Source: CAD feature listing. Evaluate the final solid. Frame: model axes, mm. Face numbers are marked on the shaded views. A direction names the side the tool comes from. Round coordinates to 2 decimals unless told otherwise and drop trailing zeros. Loops run counter-clockwise (first coordinate to the right, second up) from the corner with the lowest first, then second, coordinate; pieces in that order, holes last. Notation, with made-up numbers: M 62,73.25 L 75,73.25 A32 ccw 75,112.25 Z; hole C 32.5,75 d11. An arc over 180 degrees is marked long. Answer as a JSON object with one key per item and string values.
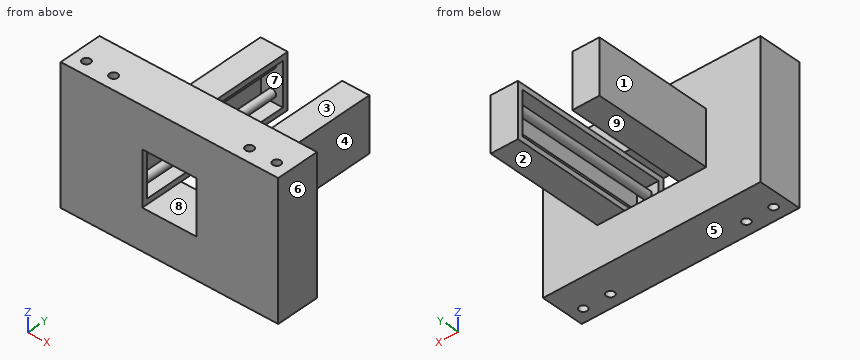
from build123d import *

# Parameters (mm, degrees)
SKETCH1_W           = 400
SKETCH1_H           = 250
BOSS_EXTRUDE1_DEPTH = 80
SKETCH2_R           = 7.5
CUT_EXTRUDE1_DEPTH  = 479.434948556
SKETCH5_W           = 200
SKETCH5_H           = 100
CUT_EXTRUDE2_DEPTH  = 479.434948556
SKETCH8_W           = 100
SKETCH8_H           = 300
BOSS_EXTRUDE2_DEPTH = 50
SKETCH9_W           = 80
SKETCH9_H           = 280
CUT_EXTRUDE3_DEPTH  = 40
SKETCH10_R          = 7.5
BOSS_EXTRUDE3_DEPTH = 280


with BuildPart() as part:
    # Sketch1 → Boss-Extrude1 (new body)
    with BuildSketch(Plane(origin=(0, 0, 0), x_dir=(1, 0, 0), z_dir=(0, 1, 0))):
        with Locations((-200, 125)):
            Rectangle(SKETCH1_W, SKETCH1_H)
    extrude(amount=BOSS_EXTRUDE1_DEPTH)

    # Sketch2 → Cut-Extrude1 (cut, through all)
    with BuildSketch(Plane.XY):
        with Locations((-375, 25)):
            Circle(SKETCH2_R)
        with Locations((-325, 25)):
            Circle(SKETCH2_R)
        with Locations((-75, 25)):
            Circle(SKETCH2_R)
        with Locations((-25, 25)):
            Circle(SKETCH2_R)
    extrude(amount=-CUT_EXTRUDE1_DEPTH, mode=Mode.SUBTRACT)

    # Sketch5 → Cut-Extrude2 (cut, through all)
    with BuildSketch(Plane(origin=(0, 80, 0), x_dir=(1, 0, 0), z_dir=(0, 1, 0))):
        with Locations((-200, 125)):
            Rectangle(SKETCH5_W, SKETCH5_H)
    extrude(amount=-CUT_EXTRUDE2_DEPTH, mode=Mode.SUBTRACT)

    # Sketch8 → Boss-Extrude2 (add)
    with BuildSketch(Plane(origin=(-300, 0, 0), x_dir=(0, 0, -1), z_dir=(1, 0, 0))):
        with Locations((125, 150)):
            Rectangle(SKETCH8_W, SKETCH8_H)
    boss_extrude2 = extrude(amount=BOSS_EXTRUDE2_DEPTH)

    # Sketch9 → Cut-Extrude3 (cut)
    with BuildSketch(Plane(origin=(-250, 0, 0), x_dir=(0, 0, -1), z_dir=(1, 0, 0))):
        with Locations((125, 150)):
            Rectangle(SKETCH9_W, SKETCH9_H)
    cut_extrude3 = extrude(amount=-CUT_EXTRUDE3_DEPTH, mode=Mode.SUBTRACT)

    # Mirror1: Boss-Extrude2, Cut-Extrude3 across plane
    add(boss_extrude2.mirror(Plane.ZY.offset(200)))
    add(cut_extrude3.mirror(Plane.ZY.offset(200)), mode=Mode.SUBTRACT)

    # Sketch10 → Boss-Extrude3 (add)
    with BuildSketch(Plane(origin=(0, 10, 0), x_dir=(1, 0, 0), z_dir=(0, 1, 0))):
        with Locations(Location((-270, 150, 0), (0, 0, 90))):
            Circle(SKETCH10_R)
        with Locations(Location((-270, 100, 0), (0, 0, 90))):
            Circle(SKETCH10_R)
    boss_extrude3 = extrude(amount=BOSS_EXTRUDE3_DEPTH)

    # Mirror2: Boss-Extrude3 across plane
    add(boss_extrude3.mirror(Plane.ZY.offset(200)))


solid = part.part
Item 1: Section B-B on y = 73.5. Return the cut outline in (x, z).
Answer sheet:
{"outline": "M -400,-250 L 0,-250 L 0,0 L -400,0 Z; C -270,-150 d15; C -270,-100 d15; C -130,-150 d15; C -130,-100 d15; hole M -290,-165 L -250,-165 L -250,-175 L -150,-175 L -150,-165 L -110,-165 L -110,-85 L -150,-85 L -150,-75 L -250,-75 L -250,-85 L -290,-85 Z"}
Item 2: Access query for the marked faces 1, 2, 3, 4 and 5. Directions: +Z, -Z, +X, -X, +Y, -Y. A direction counts if a zero-diameter tool reaches every point of the face in a straight line with its end or side. Return the directions, or none.
Answer sheet:
{"face 1": "+Z, -Z, -X, +Y", "face 2": "-Z, +X, -X, +Y", "face 3": "+Z, +X, -X, +Y", "face 4": "+Z, -Z, +X, +Y", "face 5": "-Z, +X, -X, +Y, -Y"}
Item 3: Section A-A on z = -100. Give the number of separate pieces and of enclosed holes in the cut face, then the cut area to 3 significant figures.
Answer sheet:
{"separate pieces": "2", "enclosed holes": "6", "area": "31,300 mm²"}
Item 4: Line query: probe 1 along Z at (x, y) = (-271, 39); probe 2 along X at (y, z) = (76, -100.5); probe 3 along Y at (x, z) = (-325, -72.5). Output: solid intervals per line, ascending. Write a range as from..to.
Answer sheet:
{"probe 1": "z = -250..-165, -157.43..-142.57, -107.43..-92.57, -85..0", "probe 2": "x = -400..-290, -277.48..-262.52, -137.48..-122.52, -110..0", "probe 3": "y = 0..17.5, 32.5..80"}
Item 5: Section D-D on x = -325. Return the cut outline in (y, z), then the cut area to 4 significant figures.
Answer sheet:
{"outline": "M 0,-250 L 17.5,-250 L 17.5,0 L 0,0 Z; M 32.5,-250 L 80,-250 L 80,0 L 32.5,0 Z", "area": "16,250 mm²"}
Item 6: Section C-C on y = 240.5. Return the cut outline in (x, z).
Answer sheet:
{"outline": "M -300,-175 L -250,-175 L -250,-165 L -290,-165 L -290,-85 L -250,-85 L -250,-75 L -300,-75 Z; C -270,-150 d15; C -270,-100 d15; M -150,-175 L -100,-175 L -100,-75 L -150,-75 L -150,-85 L -110,-85 L -110,-165 L -150,-165 Z; C -130,-150 d15; C -130,-100 d15"}
Item 7: Contact query for flat-ended pins moving along their axis: pin 1 Ø9 at (x, y) = (-325, 25) entering from -Z; pin 2 Ø15 at (x, y) = (-272.5, 208.5) entering from -Z; pin 3 Ø12 at (x, y) = (-304, 117.5) entering from +Z; pin 4 Ø8 at (y, z) = (263, -99) entering from -X. Output: stop coordinate, or through.
Answer sheet:
{"pin 1": "passes through", "pin 2": "stops at z = -175", "pin 3": "stops at z = -75", "pin 4": "stops at x = -300"}
Item 8: Pull-direction query (Z, two-part tool) for the marked faces 6, 7, 8 and 9; classes: pulls with the +Z half, pulls with the -Z half, needs draft (parallel to the pull), parting line crosses it, or undercut.
Answer sheet:
{"face 6": "needs draft", "face 7": "undercut", "face 8": "undercut", "face 9": "pulls with the -Z half"}
